Design review of the part built by this model. Coordinates are the model's own, in mm. A direction names the side the tool comes from. Give positions to 0.01 mm unless a question says otherwise; leave off trailing zeros. Loops run counter-clockwise (first coordinate to the right, second up) from the corner with the lowest first, then second, coordinate; pieces in that order, holes last. Notation, with made-up numbers: M 82,60 L 124,60 A18 ccw 124,87 Z; hole C 30.5,56.25 d4. An arc over 180 degrees is marked long. Use a Markdown table: item, result. Add a question column.
(1) Insertion check: pin 1 Ø3 at (x, y) = (-52, 6) entering from -Z; pin 2 Ø3 at (y, z) = (4, -7.5) entering from +X. Each pin has a flat end and moves straight along its axis. Give the tip position at first contact, or say it passes through.
(2) For faces 1 (the face through (-66, 4, -16.023)), 2 (the face through (-49.95, 8.145, -4.1)), list the 3-axis set-ups (+Z, -Z, +X, -X, +Y, -Y) from which the entire face can be reached by the end or side of a thin tool; tool diameter is ignored.
(3) Add section B-B, the plane y = 6. Give the boundary of the cut face in (x, z), then the cut area to 4 significant figures.
(4) Add section D-D, the plane x = -52.5. Give the boundary of the cut face in (y, z).
(5) For probe 1 along X at (y, z) = (4.5, -12.5); probe 2 along Y at (x, z) = (-56.5, -12.75); probe 3 along Z at (x, y) = (-48.5, 4.5), list the stretches that pass through material, from the lowest coordinate up.
(6) Add section A-A, the plane x = -69.5. Give the boundary of the cut face in (y, z), then the cut area to 3 significant figures.
(7) Add section C-C, the plane z = -13.5. Give the boundary of the cut face in (x, y), then the cut area to 3 significant figures.
(8) Draft analysis for pull direction Y (two halves, no side actions). For faces 3 (the face through (-57.345, 6, -9)), 4 (the face through (-66, 12, -9)), 5 (the face through (-66, 4, -2.523)), 6 (the face through (-49.95, 2.958, -5.305)), state which applies: pulls with the +Y half, pulls with the -Y half, needs draft (parallel to the pull), parting line crosses it, or undercut.
```python
from build123d import *

# Parameters (mm, degrees)
SKETCH1_W           = 17
SKETCH1_H           = 13.5
BOSS_EXTRUDE1_DEPTH = 12
SKETCH2_R           = 5.6
SKETCH2_R_2         = 5
BOSS_EXTRUDE2_DEPTH = 15
FILLET1_R           = 4


with BuildPart() as part:
    # Sketch1 → Boss-Extrude1 (new body)
    with BuildSketch(Plane(origin=(0, 0, 0), x_dir=(1, 0, 0), z_dir=(0, 1, 0))):
        with Locations((-65.845078181, 9.272756488)):
            Rectangle(SKETCH1_W, SKETCH1_H)
    extrude(amount=BOSS_EXTRUDE1_DEPTH)

    # Sketch2 → Boss-Extrude2 (add)
    with BuildSketch(Plane(origin=(-57.345078181, 0, 0), x_dir=(0, 0, -1), z_dir=(1, 0, 0))):
        with Locations(Location((9.272756488, 6, 0), (0, 0, 180))):
            Circle(SKETCH2_R)
        with Locations((9.272756488, 6)):
            Circle(SKETCH2_R_2, mode=Mode.SUBTRACT)
    extrude(amount=BOSS_EXTRUDE2_DEPTH)

    # Fillet1
    fillet1_edges = [part.edges().sort_by_distance(p)[0] for p in [
        (-65.845078181, 12, -16.022756488),
        (-65.845078181, 12, -2.522756488),
    ]]
    fillet(fillet1_edges, radius=FILLET1_R)


solid = part.part
```
Established:
| question | item | result |
|---|---|---|
| 1 | pin 1 | z = -14.87 |
| 1 | pin 2 | x = -57.35 |
| 2 | face 1 | -Z, +X, -X, +Y, -Y |
| 2 | face 2 | +X |
| 3 | outline | M -74.35,-16.02 L -57.35,-16.02 L -57.35,-14.87 L -42.35,-14.87 L -42.35,-14.27 L -57.35,-14.27 L -57.35,-4.27 L -42.35,-4.27 L -42.35,-3.67 L -57.35,-3.67 L -57.35,-2.52 L -74.35,-2.52 Z |
| 3 | area | 247.5 mm^2 |
| 4 | outline | C 6,-9.27 d11.2; hole C 6,-9.27 d10 |
| 5 | probe 1 | -74.35 to -57.35 |
| 5 | probe 2 | 1.61 to 2.41, 9.59 to 10.39 |
| 5 | probe 3 | -14.67 to -14.04, -4.5 to -3.88 |
| 6 | outline | M 0,-16.02 L 8,-16.02 A4 ccw 12,-12.02 L 12,-6.52 A4 ccw 8,-2.52 L 0,-2.52 Z |
| 6 | area | 155 mm^2 |
| 7 | outline | M -74.35,0 L -57.35,0 L -57.35,2.33 L -42.35,2.33 L -42.35,3.33 L -57.35,3.33 L -57.35,8.67 L -42.35,8.67 L -42.35,9.67 L -57.35,9.67 L -57.35,11.72 L -74.35,11.72 Z |
| 7 | area | 229 mm^2 |
| 8 | face 3 | undercut |
| 8 | face 4 | pulls with the +Y half |
| 8 | face 5 | needs draft |
| 8 | face 6 | undercut |
